Verification items for this drawing (mm, ordinates from the low corner). A direction names the side the tool comes from. Give positions to 0.01 mm unless a question says otherwise; leave off trailing zeros. Loops run counter-clockwise (first coordinate to the right, second up) from the corner with the lowest first, then second, coordinate; pieces in that order, holes last. Notation, with made-up numbers: (77, 27) -> (126, 27) arc R15 ccw to (126, 47) -> close; hole circle Ø10 at (-27.75, 32). An arc over 180 degrees is marked (long way). Write each question's results on one line, items separated by ' | '. Start each with the question number.
Item 1: Mould release check, pull along Z, two halves, no side actions. Record for the marked faces 1, 2 and 3: pulls with the +Z half, pulls with the -Z half, needs draft (parallel to the pull), parting line crosses it, or undercut.
Item 2: Cross-section at A-A on z = 17.5. Enter the section's corners in (x, y), then the cut area to 3 significant figures.
Item 3: Cross-section at D-D on y = 4.75. Enter the section's corners in (x, z) (1 decimal), then the cut area to 3 significant figures.
Item 4: Scan lines: line 1 along Z through (x, y) = (12, 11.75); line 2 along Z through (x, y) = (30, 21.25); line 3 along Y through (x, z) = (8.5, 24). Record each from-to range of solid material in increasing order.
Item 5: Gauge pin test, flat ends, axial feed: pin 1 Ø6 at (y, z) = (19.5, 4.5) entering from +X (1 decimal); pin 2 Ø4 at (x, y) = (60, 14.5) entering from +Z; pin 3 Ø10.5 at (x, y) = (61.5, 7.5) entering from -Z; pin 4 Ø12 at (x, z) = (30, 17.5) entering from +Y. Record the tip position at first contact, or that the pin passes through.
Item 6: Cross-section at C-C on x = 8. Enter the section's corners in (y, z).
Item 7: Cross-section at B-B on x = 30. Enter the section's corners in (y, z), then the cut area to 3 significant figures.
Item 8: Access from +Z, -Z, +X, -X, +Y, -Y to the whole of each face (thin tool, end or side, straight path). Record for the marked faces 4, 5, 6 and 7.
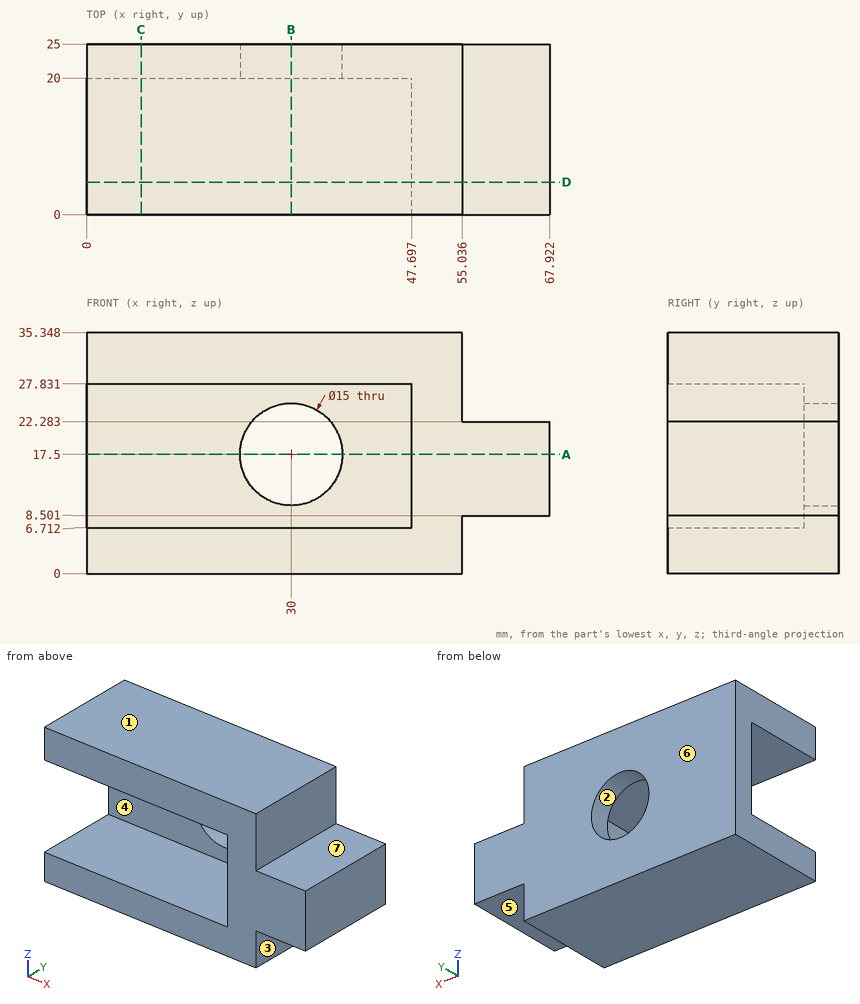
Answer sheet:
1) face 1: pulls with the +Z half | face 2: undercut | face 3: needs draft
2) outline: (0, 20) -> (22.5, 20) -> (22.5, 25) -> (0, 25) -> close; (37.5, 20) -> (47.7, 20) -> (47.7, 0) -> (67.92, 0) -> (67.92, 25) -> (37.5, 25) -> close | area: 669 mm²
3) outline: (0, 0) -> (55, 0) -> (55, 8.5) -> (67.9, 8.5) -> (67.9, 22.3) -> (55, 22.3) -> (55, 35.3) -> (0, 35.3) -> (0, 27.8) -> (47.7, 27.8) -> (47.7, 6.7) -> (0, 6.7) -> close | area: 1,120 mm²
4) line 1: z = 0 to 6.71, 27.83 to 35.35 | line 2: z = 0 to 10, 25 to 35.35 | line 3: y = 20 to 25
5) pin 1: stops at x = 55 | pin 2: stops at z = 22.28 | pin 3: stops at z = 8.5 | pin 4: passes through
6) outline: (0, 0) -> (25, 0) -> (25, 35.35) -> (0, 35.35) -> (0, 27.83) -> (20, 27.83) -> (20, 6.71) -> (0, 6.71) -> close
7) outline: (0, 0) -> (25, 0) -> (25, 10) -> (20, 10) -> (20, 6.71) -> (0, 6.71) -> close; (0, 27.83) -> (20, 27.83) -> (20, 25) -> (25, 25) -> (25, 35.35) -> (0, 35.35) -> close | area: 386 mm²
8) face 4: -X, -Y | face 5: -Z, +X, +Y, -Y | face 6: +Z, -Z, +X, -X, +Y | face 7: +Z, +X, +Y, -Y
